Verification items for the finished model (mm, model axes). Round coordinates to 2 decimals unless told otherwise and drop trailing zeros. Order: outer loops, then holes, each group sorted by start corner. A loop starts at its lowest first (then second) coordinate and runs counter-clockwise, first axis right, second up. Notation, with made-up numbers: (48, 34.5) -> (88, 34.5) arc R22 cw to (88, 67.5) -> close; hole circle Ø1 at (-31, -4.5). An arc over 180 degrees is marked (long way). Return JSON: item names as keys, results as strings. Group by question number.
1) Section check D-D on x = 7.5. Enter the section's corners in (y, z), plus the area to 3 significant figures.
2) Draft check along Y on faces 1 (the cylindrical face through (-17.01, -1.11, 2.03)), 2 (the flat face through (0, 7, 4)), 3 (the flat face through (-13.944, -14.34, 1.972)). Enter one of: pulls with the +Y half, pulls with the -Y half, needs draft (parallel to the pull), parting line crosses it, or undercut.
3) Scan lines: L1, parallel to X at y = -1, z = 2.8; L2, parallel to X at y = -16, z = 1.2; L3, parallel to X at y = 16.5, z = 2.45. Record each from-to range of solid material in increasing order.
4) Section check B-B on y = -16. Enter the section's corners in (x, z), plus the area to 3 significant figures.
5) Section check A-A on z = 2.1. Enter the section's corners in (x, y), plus the area to 3 significant figures.
6) Depth check by flat-ended pin: pin 1 (1.8 mm diameter, centred on x = 0, y = 16, fed in from +Z); pin 2 (1.5 mm diameter, centred on x = 16.5, z = 1.5, fed in from +Y); pin 3 (1.5 mm diameter, centred on y = 17, z = 3.5, fed in from -X). Enter the tip coordinate at first touch or a pass-through.
Autodesk Inventor part; units mm, degrees
ref_plane "YZ Plane" through (0, 0, 0) normal (1, 0, 0) x (0, 1, 0)
ref_plane "XZ Plane" through (0, 0, 0) normal (0, 1, 0) x (-1, 0, 0)
ref_plane "XY Plane" through (0, 0, 0) normal (0, 0, 1) x (1, 0, 0)
sketch "Náčrt1" plane through (0, 0, 0) normal (0, 0, 1) x (1, 0, 0)
  line L0 (-28.2843, 0) -> (0, 28.2843)
  line L1 (0, 28.2843) -> (28.2843, 0)
  line L2 (28.2843, 0) -> (0, -28.2843)
  line L3 (0, -28.2843) -> (-28.2843, 0)
  line L4 (-28.2843, 0) -> (28.2843, 0) construction
  line L5 (0, 28.2843) -> (0, -28.2843) construction
  line L6 (-28.2843, 0) -> (11.7157, 0) construction
  line L7 (0, 39.598) -> (0, -39.598)
  line L8 (-39.598, 0) -> (39.598, 0)
  point P0 (0, 0)
  point P1 (-16, 0)
  point P2 (16, 0)
  point P3 (0, 0)
  point P4 (0, 16)
  point P5 (0, -16)
  point P6 (0, 0)
  point P7 (0, 0)
  dimension "d0" = 40
  dimension "d2" = 40
  dimension "d3" = 32
  dimension "d4" = 16
  dimension "d5" = 32
  dimension "d6" = 16
  dimension "d9" = 90
  dimension "d10" = 90
extrude "Vysunutí1" add sketch "Náčrt1" along normal blind 4
hole "Díra1" at (-16, 0, 0) at (16, 0, 0) at (0, 16, 0) at (0, -16, 0) direction (0, 0, 1) diameter 3 end through all
hole "Díra2" at (0, 0, 0) direction (0, 0, 1) diameter 6 end through all
properties part number "drzakmotoru_nový"
Check result:
{
 "1": {"outline": "(-20.78, 0) -> (20.78, 0) -> (20.78, 4) -> (-20.78, 4) -> close", "area": "166 mm^2"},
 "2": {"face 1": "undercut", "face 2": "needs draft", "face 3": "pulls with the -Y half"},
 "3": {"L1": "-27.28 to -17.12, -14.88 to -2.83, 2.83 to 14.88, 17.12 to 27.28", "L2": "-12.28 to -1.5, 1.5 to 12.28", "L3": "-11.78 to -1.41, 1.41 to 11.78"},
 "4": {"outline": "(-12.28, 0) -> (-1.5, 0) -> (-1.5, 4) -> (-12.28, 4) -> close; (1.5, 0) -> (12.28, 0) -> (12.28, 4) -> (1.5, 4) -> close", "area": "86.3 mm^2"},
 "5": {"outline": "(-28.28, 0) -> (0, -28.28) -> (28.28, 0) -> (0, 28.28) -> close; hole circle Ø3 at (-16, 0); hole circle Ø6 at (0, 0); hole circle Ø3 at (0, -16); hole circle Ø3 at (0, 16); hole circle Ø3 at (16, 0)", "area": "1,540 mm^2"},
 "6": {"pin 1": "through", "pin 2": "y = 12.53", "pin 3": "x = -12.03"}
}
